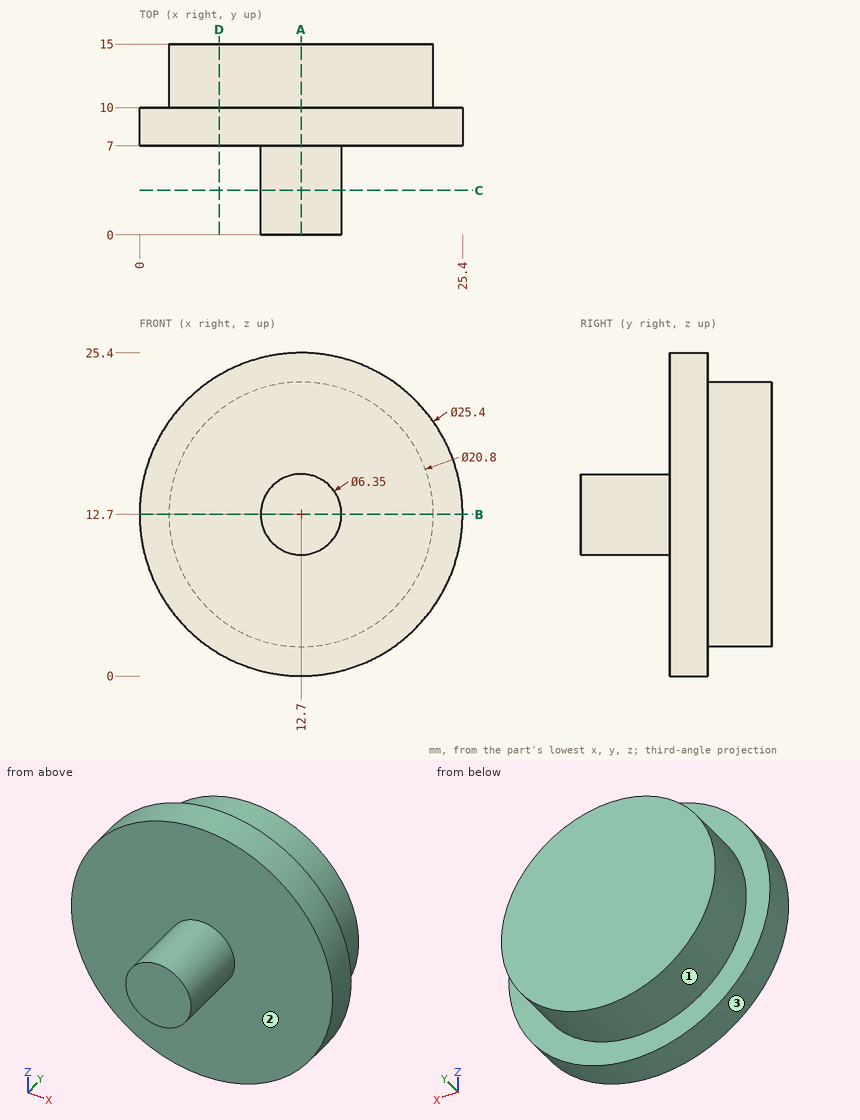
The figure shows three views and two pictorial views of one solid part (mm, origin at its lowest corner). Answer the questions. A direction names the side the tool comes from. Give positions to 0.01 mm unless a question says otherwise; leave off trailing zeros. Write each loop counter-clockwise with the first axis right and the second up, starting at its lowest first coordinate (ties: lowest second). Pieces come first, ordered by that corner, then holes. Notation, with made-up numbers: M -7.5,86 L 17.5,86 A25 cw 17.5,118 Z; hole C 34,42 d5. An arc over 180 degrees is marked long. One line per item, written item: value. Start each with the question number.
(1) Flat-ended cylindrical pins translate along their axes: pin 1 Ø4 at (x, z) = (15.5, 7) entering from -Y; pin 2 Ø8 at (y, z) = (10, 18) entering from -X; pin 3 Ø1.5 at (x, y) = (8, 11.5) entering from -Z. Find the tip coordinate at first contact, or state that the pin passes through.
(2) A tool of negligible diameter and unlimited length cuts with its end or side. For the marked faces 1, 2 and 3, from which of +Z, -Z, +X, -X, +Y, -Y can it reach the whole face along a straight path? Write none if from no direction.
(3) Find the intervals of material crossed by line 1 (Y direction, x = 12.25, z = 5.25); line 2 (Y direction, x = 5, z = 4.25); line 3 (X direction, y = 10.75, z = 3.5), in increasing order.
(4) Find section C-C (y = 3.5). Determine the outline of the cut face in (x, z) (3 decimals).
(5) Find section D-D (x = 6.25). Determine the outline of the cut face in (y, z).
(6) Find section A-A (x = 12.7). Determine the outline of the cut face in (y, z) (3 decimals), plus the area to 3 significant figures.
(7) Find section B-B (z = 12.7). Determine the outline of the cut face in (x, y) (3 decimals), plus the area to 3 significant figures.
Results below:
1. pin 1: stops at y = 7
1. pin 2: stops at x = 0.07
1. pin 3: stops at z = 3.08
2. face 1: +Y
2. face 2: -Y
2. face 3: +Y, -Y
3. line 1: y = 7 to 15
3. line 2: y = 7 to 10
3. line 3: x = 7.85 to 17.55
4. outline: C 12.7,12.7 d6.35
5. outline: M 7,1.76 L 10,1.76 L 10,4.54 L 15,4.54 L 15,20.86 L 10,20.86 L 10,23.64 L 7,23.64 Z
6. outline: M 0,9.525 L 7,9.525 L 7,0 L 10,0 L 10,2.3 L 15,2.3 L 15,23.1 L 10,23.1 L 10,25.4 L 7,25.4 L 7,15.875 L 0,15.875 Z
6. area: 225 mm^2
7. outline: M 0,7 L 9.525,7 L 9.525,0 L 15.875,0 L 15.875,7 L 25.4,7 L 25.4,10 L 23.1,10 L 23.1,15 L 2.3,15 L 2.3,10 L 0,10 Z
7. area: 225 mm^2
